```python
from build123d import *

# Parameters (mm, degrees)
F0_R     = 25.4
F1_DEPTH = 76.2
F2_W     = 20.5636313185
F2_H     = 12.2810583562
F3_DEPTH = 76.2
F5_DEPTH = 76.2


with BuildPart() as f1:
    # F0 (on Front) → F1 (new body)
    with BuildSketch(Plane.XZ):
        Circle(F0_R)
    extrude(amount=F1_DEPTH)

    # F2 (on face) → F3 (cut)
    with BuildSketch(Plane.XZ.offset(76.2)):
        with Locations((-19.2842693068, 21.6356487945)):
            Rectangle(F2_W, F2_H)
    extrude(amount=-F3_DEPTH, mode=Mode.SUBTRACT)

    # F4 (on face) → F5 (cut)
    with BuildSketch(Plane.XZ.offset(76.2)):
        with BuildLine():
            Line((12.1693527326, 12.8687405959), (3.7766969763, 12.8687405959))
            ThreePointArc((3.7766969763, 12.8687405959), (7.9730248544, 9.231923148), (12.1693527326, 12.8687405959))
        make_face()
        with BuildLine():
            Line((3.7766969763, 14.0738399925), (3.7766969763, 12.8687405959))
            Line((3.7766969763, 12.8687405959), (12.1693527326, 12.8687405959))
            Line((12.1693527326, 12.8687405959), (12.1693527326, 14.0738399925))
            ThreePointArc((12.1693527326, 14.0738399925), (7.9730248544, 17.7106574404), (3.7766969763, 14.0738399925))
        make_face()
        with BuildLine():
            Line((3.7766969763, 36.0884256661), (3.7766969763, 25.1176543481))
            ThreePointArc((3.7766969763, 25.1176543481), (8.096973208, 24.0748629252), (12.1693527326, 22.2949961666))
            Line((12.1693527326, 22.2949961666), (12.1693527326, 36.0884256661))
            Line((12.1693527326, 36.0884256661), (3.7766969763, 36.0884256661))
        make_face()
        with BuildLine():
            Line((3.7766969763, 25.1176543481), (3.7766969763, 14.0738399925))
            ThreePointArc((3.7766969763, 14.0738399925), (7.9730248544, 17.7106574404), (12.1693527326, 14.0738399925))
            Line((12.1693527326, 14.0738399925), (12.1693527326, 22.2949961666))
            ThreePointArc((12.1693527326, 22.2949961666), (8.096973208, 24.0748629252), (3.7766969763, 25.1176543481))
        make_face()
    extrude(amount=-F5_DEPTH, mode=Mode.SUBTRACT)


solid = f1.part
```
Input: part model. Units: mm. Frame: model coordinates. A direction names the side the tool comes from. Coordinates: 2 decimals unless noted, no trailing zeros. Write each loop counter-clockwise with the first axis right and the second up, starting at its lowest first coordinate (ties: lowest second). Pieces come first, ordered by that corner, then holes. Notation, with made-up numbers: M -20,16.25 L 15,16.25 A32 ccw 15,51.25 Z; hole C 54.5,41 d5. An arc over 180 degrees is marked long. Use one line per item in the form item = value.
Q1. Section C-C (x = 15). Return loops of the section in (y, z), plus the area to 3 significant figures.
Answer below:
outline = M -76.2,-20.5 L 0,-20.5 L 0,20.5 L -76.2,20.5 Z
area = 3,120 mm²
Q2. Draft query along X for faces 1 (the face through (12.169, -39, 18)), 2 (the face through (-15, -39, 15.495)), 3 (the face through (-9.002, -39, 20)), 4 (the face through (7.888, -38.633, 9.233)). Return one class per face: released by +X, released by -X, zero draft, split by the parting line, or undercut.
Answer below:
face_1 = undercut
face_2 = zero draft
face_3 = released by -X
face_4 = undercut
Q3. Material intervals for probe 1 along X at (y, z) = (-8, 22); probe 2 along X at (y, z) = (-28, 12.5); probe 3 along Z at (x, y) = (0.5, -32), sorted ascending. Write a range as from..to.
Answer below:
probe_1 = -9..3.78, 12.17..12.69
probe_2 = -22.11..3.85, 12.1..22.11
probe_3 = -25.4..25.4
Q4. First-contact query: pin 1 (10.5 mm diameter, centred on y = -37, z = 16, fed in from -X); pin 2 (5 mm diameter, centred on y = -30.5, z = -18.5, fed in from +X); pin 3 (10 mm diameter, centred on y = -65.5, z = -10.5, fed in from -X). Flat tips, straight axial feed; report the tip coordinate or a pass-through.
Answer below:
pin_1 = -23.01
pin_2 = 19.73
pin_3 = -24.8
Q5. Set-up query: faces 5 (the face through (0, -76.2, 0)), 6 (the face through (3.777, -39, 19)). Return all of +Z, -Z, +X, -X, +Y, -Y with unobstructed straight access to the full face (end or side cutting, diameter ignored); none if empty.
Answer below:
face_5 = +Z, -Z, +X, -X, -Y
face_6 = +Z, +Y, -Y
Q6. Section A-A (z = 19). Return loops of the section in (x, y).
Answer below:
outline = M -9,-76.2 L 3.78,-76.2 L 3.78,0 L -9,0 Z; M 12.17,-76.2 L 16.86,-76.2 L 16.86,0 L 12.17,0 Z
Q7. Section D-D (z = 6). Return loops of the section in (x, y), plus the area to 3 significant figures.
Answer below:
outline = M -24.68,-76.2 L 24.68,-76.2 L 24.68,0 L -24.68,0 Z
area = 3,760 mm²
Q8. Section B-B (y = -68). Return loops of the section in (x, z) (3 decimals), plus the area to 3 significant figures.
Answer below:
outline = M -20.126,15.495 A25.4 ccw long 12.169,22.295 L 12.169,12.869 A4.239 cw 3.777,12.869 L 3.777,25.118 A25.4 ccw -9.002,23.751 L -9.002,15.495 Z
area = 1,860 mm²
